Source: CAD feature listing. Evaluate the final solid. Frame: model axes, mm. Round coordinates to 2 decimals unless told otherwise and drop trailing zeros. Loops run counter-clockwise (first coordinate to the right, second up) from the corner with the lowest first, then second, coordinate; pieces in that order, holes last. Notation, with made-up numbers: M 8.25,-33 L 55.25,-33 A24 cw 55.25,-15 Z; hole C -37,50 d8. An arc over 180 degrees is marked long. One line per item, written item: value.
from build123d import *

# Parameters (mm, degrees)
F0_W     = 5
F0_H     = 5
F1_DEPTH = 4


with BuildPart() as f1:
    # F0 (on Top) → F1 (new body)
    with BuildSketch(Plane.XY):
        with BuildLine():
            Line((82.7990943193, -150.3260023594), (82.7990943193, -150.8260023594))
            Line((82.7990943193, -150.8260023594), (85.2990943193, -150.8260023594))
            Line((85.2990943193, -150.8260023594), (85.2990943193, -148.3260023594))
            Line((85.2990943193, -148.3260023594), (84.7990943193, -148.3260023594))
            ThreePointArc((84.7990943193, -148.3260023594), (84.2133078817, -149.7402159218), (82.7990943193, -150.3260023594))
        make_face()
        with BuildLine():
            Line((-45.2009056807, -148.3260023594), (-45.7009056807, -148.3260023594))
            Line((-45.7009056807, -148.3260023594), (-45.7009056807, -150.8260023594))
            Line((-45.7009056807, -150.8260023594), (-43.2009056807, -150.8260023594))
            Line((-43.2009056807, -150.8260023594), (-43.2009056807, -150.3260023594))
            ThreePointArc((-43.2009056807, -150.3260023594), (-44.615119243, -149.7402159218), (-45.2009056807, -148.3260023594))
        make_face()
        with BuildLine():
            Line((-43.2009056807, 49.1739976406), (-43.2009056807, 49.6739976406))
            Line((-43.2009056807, 49.6739976406), (-45.7009056807, 49.6739976406))
            Line((-45.7009056807, 49.6739976406), (-45.7009056807, 47.1739976406))
            Line((-45.7009056807, 47.1739976406), (-45.2009056807, 47.1739976406))
            ThreePointArc((-45.2009056807, 47.1739976406), (-44.615119243, 48.588211203), (-43.2009056807, 49.1739976406))
        make_face()
        with BuildLine():
            Line((85.2990943193, -61.3260023594), (85.2990943193, -58.8260023594))
            Line((85.2990943193, -58.8260023594), (82.7990943193, -58.8260023594))
            Line((82.7990943193, -58.8260023594), (82.7990943193, -59.3260023594))
            ThreePointArc((82.7990943193, -59.3260023594), (84.2133078817, -59.911788797), (84.7990943193, -61.3260023594))
            Line((84.7990943193, -61.3260023594), (85.2990943193, -61.3260023594))
        make_face()
        with BuildLine():
            Line((19.2990943193, 49.6739976406), (16.7990943193, 49.6739976406))
            Line((16.7990943193, 49.6739976406), (16.7990943193, 49.1739976406))
            ThreePointArc((16.7990943193, 49.1739976406), (18.2133078817, 48.588211203), (18.7990943193, 47.1739976406))
            Line((18.7990943193, 47.1739976406), (19.2990943193, 47.1739976406))
            Line((19.2990943193, 47.1739976406), (19.2990943193, 49.6739976406))
        make_face()
        with BuildLine():
            Line((85.2990943193, -63.8260023594), (85.2990943193, -61.3260023594))
            Line((85.2990943193, -61.3260023594), (84.7990943193, -61.3260023594))
            ThreePointArc((84.7990943193, -61.3260023594), (81.384880757, -62.7402159218), (82.7990943193, -59.3260023594))
            Line((82.7990943193, -59.3260023594), (82.7990943193, -58.8260023594))
            Line((82.7990943193, -58.8260023594), (80.2990943193, -58.8260023594))
            Line((80.2990943193, -58.8260023594), (80.2990943193, -63.8260023594))
            Line((80.2990943193, -63.8260023594), (85.2990943193, -63.8260023594))
        make_face()
        with BuildLine():
            Line((14.2990943193, 49.6739976406), (14.2990943193, 44.6739976406))
            Line((14.2990943193, 44.6739976406), (16.7990943193, 44.6739976406))
            Line((16.7990943193, 44.6739976406), (19.2990943193, 44.6739976406))
            Line((19.2990943193, 44.6739976406), (19.2990943193, 47.1739976406))
            Line((19.2990943193, 47.1739976406), (18.7990943193, 47.1739976406))
            ThreePointArc((18.7990943193, 47.1739976406), (15.384880757, 45.7597840782), (16.7990943193, 49.1739976406))
            Line((16.7990943193, 49.1739976406), (16.7990943193, 49.6739976406))
            Line((16.7990943193, 49.6739976406), (14.2990943193, 49.6739976406))
        make_face()
        with BuildLine():
            Line((-37.7009056807, -58.8260023594), (-40.7009056807, -58.8260023594))
            Line((-40.7009056807, -58.8260023594), (-40.7009056807, -52.8260023594))
            Line((-40.7009056807, -52.8260023594), (-40.7009056807, 28.4739976406))
            Line((-40.7009056807, 28.4739976406), (-40.7009056807, 44.6739976406))
            Line((-40.7009056807, 44.6739976406), (14.2990943193, 44.6739976406))
            Line((14.2990943193, 44.6739976406), (14.2990943193, 49.6739976406))
            Line((14.2990943193, 49.6739976406), (-43.2009056807, 49.6739976406))
            Line((-43.2009056807, 49.6739976406), (-43.2009056807, 49.1739976406))
            ThreePointArc((-43.2009056807, 49.1739976406), (-41.7866921183, 48.588211203), (-41.2009056807, 47.1739976406))
            ThreePointArc((-41.2009056807, 47.1739976406), (-43.2009056807, 45.1739976406), (-45.2009056807, 47.1739976406))
            Line((-45.2009056807, 47.1739976406), (-45.7009056807, 47.1739976406))
            Line((-45.7009056807, 47.1739976406), (-45.7009056807, -148.3260023594))
            Line((-45.7009056807, -148.3260023594), (-45.2009056807, -148.3260023594))
            ThreePointArc((-45.2009056807, -148.3260023594), (-43.2009056807, -146.3260023594), (-41.2009056807, -148.3260023594))
            ThreePointArc((-41.2009056807, -148.3260023594), (-41.7866921183, -149.7402159218), (-43.2009056807, -150.3260023594))
            Line((-43.2009056807, -150.3260023594), (-43.2009056807, -150.8260023594))
            Line((-43.2009056807, -150.8260023594), (82.7990943193, -150.8260023594))
            Line((82.7990943193, -150.8260023594), (82.7990943193, -150.3260023594))
            ThreePointArc((82.7990943193, -150.3260023594), (81.384880757, -146.911788797), (84.7990943193, -148.3260023594))
            Line((84.7990943193, -148.3260023594), (85.2990943193, -148.3260023594))
            Line((85.2990943193, -148.3260023594), (85.2990943193, -63.8260023594))
            Line((85.2990943193, -63.8260023594), (80.2990943193, -63.8260023594))
            Line((80.2990943193, -63.8260023594), (80.2990943193, -58.8260023594))
            Line((80.2990943193, -58.8260023594), (68.2990943193, -58.8260023594))
            Line((68.2990943193, -58.8260023594), (68.2990943193, -22.3260023594))
            Line((68.2990943193, -22.3260023594), (63.2990943193, -22.3260023594))
            Line((63.2990943193, -22.3260023594), (53.2990943193, -22.3260023594))
            Line((53.2990943193, -22.3260023594), (53.2990943193, -25.3760023594))
            Line((53.2990943193, -25.3760023594), (53.2990943193, -27.3260023594))
            Line((53.2990943193, -27.3260023594), (51.3490943193, -27.3260023594))
            Line((51.3490943193, -27.3260023594), (28.5490943193, -27.3260023594))
            Line((28.5490943193, -27.3260023594), (19.2990943193, -27.3260023594))
            Line((19.2990943193, -27.3260023594), (19.2990943193, -25.3760023594))
            Line((19.2990943193, -25.3760023594), (19.2990943193, -2.2760023594))
            Line((19.2990943193, -2.2760023594), (19.2990943193, -0.3260023594))
            Line((19.2990943193, -0.3260023594), (14.2990943193, -0.3260023594))
            Line((14.2990943193, -0.3260023594), (14.2990943193, -27.3260023594))
            Line((14.2990943193, -27.3260023594), (14.2990943193, -32.3260023594))
            Line((14.2990943193, -32.3260023594), (14.2990943193, -47.2260023594))
            Line((14.2990943193, -47.2260023594), (14.2990943193, -58.8260023594))
            Line((14.2990943193, -58.8260023594), (11.2990943193, -58.8260023594))
            Line((11.2990943193, -58.8260023594), (-37.7009056807, -58.8260023594))
        make_face()
        Polygon((76.8990943193, -63.8260023594), (80.2990943193, -63.8260023594), (80.2990943193, -67.2260023594), (80.2990943193, -142.4260023594), (80.2990943193, -145.8260023594), (76.8990943193, -145.8260023594), (-37.3009056807, -145.8260023594), (-40.7009056807, -145.8260023594), (-40.7009056807, -142.4260023594), (-40.7009056807, -67.2260023594), (-40.7009056807, -63.8260023594), (-37.3009056807, -63.8260023594), (14.2990943193, -63.8260023594), (19.2990943193, -63.8260023594), align=None, mode=Mode.SUBTRACT)
        Polygon((53.5990943193, -58.8260023594), (19.2990943193, -58.8260023594), (19.2990943193, -32.3260023594), (53.5990943193, -32.3260023594), (55.2990943193, -32.3260023594), (55.2990943193, -34.0260023594), (55.2990943193, -57.1260023594), (55.2990943193, -58.8260023594), align=None, mode=Mode.SUBTRACT)
        with Locations((16.7990943193, 2.1739976406)):
            Rectangle(F0_W, F0_H)
        Polygon((16.7990943193, 44.6739976406), (14.2990943193, 44.6739976406), (14.2990943193, 29.8739976406), (14.2990943193, 4.6739976406), (19.2990943193, 4.6739976406), (19.2990943193, 44.6739976406), align=None)
        with BuildLine():
            Line((65.7990943193, 4.6739976406), (19.2990943193, 4.6739976406))
            Line((19.2990943193, 4.6739976406), (19.2990943193, -0.3260023594))
            Line((19.2990943193, -0.3260023594), (28.5490943193, -0.3260023594))
            Line((28.5490943193, -0.3260023594), (51.3490943193, -0.3260023594))
            Line((51.3490943193, -0.3260023594), (53.2990943193, -0.3260023594))
            Line((53.2990943193, -0.3260023594), (53.2990943193, -2.2760023594))
            Line((53.2990943193, -2.2760023594), (53.2990943193, -5.3260023594))
            Line((53.2990943193, -5.3260023594), (63.2990943193, -5.3260023594))
            Line((63.2990943193, -5.3260023594), (68.2990943193, -5.3260023594))
            Line((68.2990943193, -5.3260023594), (68.2990943193, 2.1739976406))
            Line((68.2990943193, 2.1739976406), (67.7990943193, 2.1739976406))
            ThreePointArc((67.7990943193, 2.1739976406), (64.384880757, 0.7597840782), (65.7990943193, 4.1739976406))
            Line((65.7990943193, 4.1739976406), (65.7990943193, 4.6739976406))
        make_face()
        with BuildLine():
            Line((68.2990943193, 4.6739976406), (65.7990943193, 4.6739976406))
            Line((65.7990943193, 4.6739976406), (65.7990943193, 4.1739976406))
            ThreePointArc((65.7990943193, 4.1739976406), (67.2133078817, 3.588211203), (67.7990943193, 2.1739976406))
            Line((67.7990943193, 2.1739976406), (68.2990943193, 2.1739976406))
            Line((68.2990943193, 2.1739976406), (68.2990943193, 4.6739976406))
        make_face()
    extrude(amount=-F1_DEPTH)


solid = f1.part
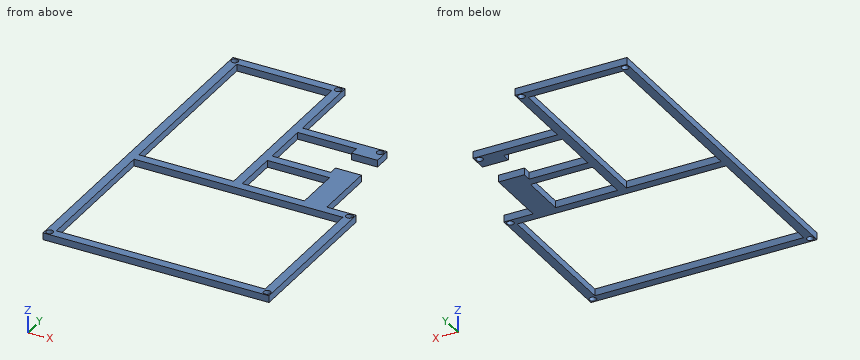
1. Section query A-A (x = 47). Return the cut outline in (y, z), and give its area (3 significant figures).
Report:
outline: M -150.83,-4 L -145.83,-4 L -145.83,0 L -150.83,0 Z; M -63.83,-4 L -58.83,-4 L -58.83,0 L -63.83,0 Z; M -32.33,-4 L -27.33,-4 L -27.33,0 L -32.33,0 Z; M -0.33,-4 L 4.67,-4 L 4.67,0 L -0.33,0 Z
area: 80.0 mm2
2. Section query D-D (z = -2.3). Count the separate pieces of the cut face and the enclosed holes in it, and give its area (3 significant figures).
Report:
separate pieces: 1
enclosed holes: 9
area: 4,400 mm2
3. Section query C-C (x = -25.5). Return the cut outline in (y, z).
Report:
outline: M -150.83,-4 L -145.83,-4 L -145.83,0 L -150.83,0 Z; M -63.83,-4 L -58.83,-4 L -58.83,0 L -63.83,0 Z; M 44.67,-4 L 49.67,-4 L 49.67,0 L 44.67,0 Z
4. Section query B-B (y = -125.5). Return the cut outline in (x, z).
Report:
outline: M -45.7,-4 L -40.7,-4 L -40.7,0 L -45.7,0 Z; M 80.3,-4 L 85.3,-4 L 85.3,0 L 80.3,0 Z
5. Ray query, line 1 (X direction, y = -52.5, z = -1.95); line 2 (Y direction, x = -1, z = -0.2); line 3 (X direction, y = -2, z = -2.45). Return the intervals inside material, ascending. Write a range as [from, to].
Report:
line 1: x = [-45.7, -40.7], [14.3, 19.3], [55.3, 68.3]
line 2: y = [-150.83, -145.83], [-63.83, -58.83], [44.67, 49.67]
line 3: x = [-45.7, -40.7], [14.3, 19.3], [53.3, 68.3]
6. Pin query (flat end, axial travel): pin 1 (3.5 mm diameter, centred on x = 82.8, y = -61.33, fed in from -Z); pin 2 (1 mm diameter, centred on y = -49.5, z = -2.5, fed in from +X). Return the tip coordinate at first contact, or that it passes through.
Report:
pin 1: passes through
pin 2: stops at x = 68.3
